Part model, mm, in its own coordinate system. Face numbers are marked on the shaded views. A direction names the side the tool comes from. Give positions to 0.01 mm unless a question says otherwise; leave off trailing zeros. Order: outer loops, then holes, each group sorted by start corner. A loop starts at its lowest first (then second) coordinate and runs counter-clockwise, first axis right, second up. Notation, with made-up numbers: (89.5, 73) - (115.5, 73) arc R12 cw to (115.5, 92) - close; hole circle Ø1 at (21.5, 89.5). An arc over 180 degrees is marked (long way). Use one line per item in the form item = value. Start each with the question number.
1. Band-saw the part on C-C, the plane z = -1.8. List the corners of the cut face in (x, y), plus the area to 3 significant figures.
2. Pull direction X, two halves, no side cores. Call the marked faces 4, 5 and 6: +X half, -X half, draft (parallel to the pull), parting line (faces both ways), or undercut.
3. Band-saw the part on D-D, the plane x = 2.3. List the corners of the cut face in (y, z).
4. Tool access for the marked faces 1, 2 and 3: list every direction of +Z, -Z, +X, -X, +Y, -Y with a clear straight run to the whole face (end or side of a thin tool).
5. Pin check, flat tips, straight feed: P1, Ø1.3, axis at x = -2, z = 0.5, coming from the +Y side; P2, Ø0.8, axis at x = 2, z = -0.5, coming from the -Y side; P3, Ø1.5, axis at y = -14, z = 0, coming from the +X side. Stop position of each tip, or through.
6. Drill centre lines: line 1 (Y direction, x = -2.2, z = -1.4); line 2 (X direction, y = 4, z = -0.15); line 3 (X direction, y = 17, z = 0.8). Where is each one in solid material? Low to high.
7. Band-saw the part on B-B, the plane y = -13. List the corners of the cut face in (x, z).
8. Band-saw the part on A-A, the plane z = 1.2. List the corners of the cut face in (x, y), plus the area to 3 significant figures.
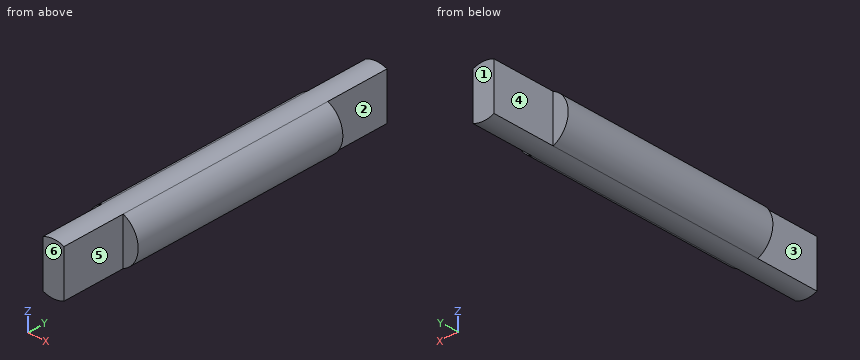
from build123d import *

# Parameters (mm, degrees)
F1_DEPTH = 18.7
F2_DEPTH = 11.85


with BuildPart() as f1:
    # F0 (on Front) → F1 (new body, symmetric)
    with BuildSketch(Plane.XZ):
        with BuildLine():
            Line((1.1339226358, -2.5053381919), (1.1339226358, 2.5053381919))
            ThreePointArc((1.1339226358, 2.5053381919), (0, 2.75), (-1.1339226358, 2.5053381919))
            Line((-1.1339226358, 2.5053381919), (-1.1339226358, -2.5053381919))
            ThreePointArc((-1.1339226358, -2.5053381919), (0, -2.75), (1.1339226358, -2.5053381919))
        make_face()
    extrude(amount=F1_DEPTH, both=True)

    # F0 (on Front) → F2 (join, symmetric)
    with BuildSketch(Plane.XZ):
        with BuildLine():
            Line((-1.1339226358, -2.5053381919), (-1.1339226358, 2.5053381919))
            ThreePointArc((-1.1339226358, 2.5053381919), (-2.75, 0), (-1.1339226358, -2.5053381919))
        make_face()
        with BuildLine():
            ThreePointArc((1.1339226358, -2.5053381919), (2.310929169, -1.4906731284), (2.75, 0))
            ThreePointArc((2.75, 0), (2.310929169, 1.4906731284), (1.1339226358, 2.5053381919))
            Line((1.1339226358, 2.5053381919), (1.1339226358, -2.5053381919))
        make_face()
    extrude(amount=F2_DEPTH, both=True)


solid = f1.part
From the geometry:
q1.outline = (-2.08, -11.85) - (-1.13, -11.85) - (-1.13, -18.7) - (1.13, -18.7) - (1.13, -11.85) - (2.08, -11.85) - (2.08, 11.85) - (1.13, 11.85) - (1.13, 18.7) - (-1.13, 18.7) - (-1.13, 11.85) - (-2.08, 11.85) - close
q1.area = 130 mm²
q2.face_4 = -X half
q2.face_5 = +X half
q2.face_6 = draft
q3.outline = (-11.85, -1.51) - (11.85, -1.51) - (11.85, 1.51) - (-11.85, 1.51) - close
q4.face_1 = +Z, -Z, +X, -X, +Y
q4.face_2 = +Z, -Z, +X, +Y
q4.face_3 = +Z, -Z, -X, -Y
q5.P1 = 11.85
q5.P2 = -11.85
q5.P3 = 1.13
q6.line_1 = -11.85 to 11.85
q6.line_2 = -2.75 to 2.75
q6.line_3 = -1.13 to 1.13
q7.outline = (-1.13, -2.51) arc R2.75 ccw to (1.13, -2.51) - (1.13, 2.51) arc R2.75 ccw to (-1.13, 2.51) - close
q8.outline = (-2.47, -11.85) - (-1.13, -11.85) - (-1.13, -18.7) - (1.13, -18.7) - (1.13, -11.85) - (2.47, -11.85) - (2.47, 11.85) - (1.13, 11.85) - (1.13, 18.7) - (-1.13, 18.7) - (-1.13, 11.85) - (-2.47, 11.85) - close
q8.area = 148 mm²
